```python
from build123d import *

# Parameters (mm, degrees)
ESBO_O1_W                = 170
ESBO_O1_H                = 96
RESSALTO_EXTRUS_O1_DEPTH = 6
CORTE_EXTRUS_O1_REACH    = 99.801
ESBO_O2_W                = 15.455454545
ESBO_O2_H                = 6
CORTE_EXTRUS_O2_REACH    = 99.801
ESBO_O3_W                = 6
ESBO_O3_H                = 13.714285714
CORTE_EXTRUS_O3_REACH    = 99.801
ESBO_O4_W                = 40
ESBO_O4_H                = 6
ESBO_O4_R                = 2.3
FILETE1_R                = 3


with BuildPart() as part:
    # Esboço1 → Ressalto-extrusão1 (new body)
    with BuildSketch(Plane(origin=(0, 0, 0), x_dir=(0, 0, -1), z_dir=(1, 0, 0))):
        Rectangle(ESBO_O1_W, ESBO_O1_H)
    extrude(amount=RESSALTO_EXTRUS_O1_DEPTH)

    # Esboço2 → Corte-extrusão1 (cut, up to next)
    with BuildSketch(Plane(origin=(6, 0, 0), x_dir=(0, 0, -1), z_dir=(1, 0, 0)), mode=Mode.PRIVATE) as corte_extrus_o1_sk1:
        with Locations((0.002272727, 45)):
            Rectangle(ESBO_O2_W, ESBO_O2_H)
    corte_extrus_o1_tool1 = extrude(corte_extrus_o1_sk1.sketch, amount=-CORTE_EXTRUS_O1_REACH, mode=Mode.PRIVATE) & part.part
    # Esboço2 → Corte-extrusão1 (cut, up to next)
    with BuildSketch(Plane(origin=(6, 0, 0), x_dir=(0, 0, -1), z_dir=(1, 0, 0)), mode=Mode.PRIVATE) as corte_extrus_o1_sk2:
        with Locations((-30.907727273, 45)):
            Rectangle(ESBO_O2_W, ESBO_O2_H)
    corte_extrus_o1_tool2 = extrude(corte_extrus_o1_sk2.sketch, amount=-CORTE_EXTRUS_O1_REACH, mode=Mode.PRIVATE) & part.part
    # Esboço2 → Corte-extrusão1 (cut, up to next)
    with BuildSketch(Plane(origin=(6, 0, 0), x_dir=(0, 0, -1), z_dir=(1, 0, 0)), mode=Mode.PRIVATE) as corte_extrus_o1_sk3:
        with Locations((-61.817727273, 45)):
            Rectangle(ESBO_O2_W, ESBO_O2_H)
    corte_extrus_o1_tool3 = extrude(corte_extrus_o1_sk3.sketch, amount=-CORTE_EXTRUS_O1_REACH, mode=Mode.PRIVATE) & part.part
    # Esboço2 → Corte-extrusão1 (cut, up to next)
    with BuildSketch(Plane(origin=(6, 0, 0), x_dir=(0, 0, -1), z_dir=(1, 0, 0)), mode=Mode.PRIVATE) as corte_extrus_o1_sk4:
        with Locations((30.912272728, 45)):
            Rectangle(ESBO_O2_W, ESBO_O2_H)
    corte_extrus_o1_tool4 = extrude(corte_extrus_o1_sk4.sketch, amount=-CORTE_EXTRUS_O1_REACH, mode=Mode.PRIVATE) & part.part
    # Esboço2 → Corte-extrusão1 (cut, up to next)
    with BuildSketch(Plane(origin=(6, 0, 0), x_dir=(0, 0, -1), z_dir=(1, 0, 0)), mode=Mode.PRIVATE) as corte_extrus_o1_sk5:
        with Locations((61.822272728, 45)):
            Rectangle(ESBO_O2_W, ESBO_O2_H)
    corte_extrus_o1_tool5 = extrude(corte_extrus_o1_sk5.sketch, amount=-CORTE_EXTRUS_O1_REACH, mode=Mode.PRIVATE) & part.part
    # Esboço2 → Corte-extrusão1 (cut, up to next)
    with BuildSketch(Plane(origin=(6, 0, 0), x_dir=(0, 0, -1), z_dir=(1, 0, 0)), mode=Mode.PRIVATE) as corte_extrus_o1_sk6:
        with Locations((-61.817727273, -48)):
            Rectangle(ESBO_O2_W, ESBO_O2_H)
    corte_extrus_o1_tool6 = extrude(corte_extrus_o1_sk6.sketch, amount=-CORTE_EXTRUS_O1_REACH, mode=Mode.PRIVATE) & part.part
    # Esboço2 → Corte-extrusão1 (cut, up to next)
    with BuildSketch(Plane(origin=(6, 0, 0), x_dir=(0, 0, -1), z_dir=(1, 0, 0)), mode=Mode.PRIVATE) as corte_extrus_o1_sk7:
        with Locations((-30.907727273, -48)):
            Rectangle(ESBO_O2_W, ESBO_O2_H)
    corte_extrus_o1_tool7 = extrude(corte_extrus_o1_sk7.sketch, amount=-CORTE_EXTRUS_O1_REACH, mode=Mode.PRIVATE) & part.part
    # Esboço2 → Corte-extrusão1 (cut, up to next)
    with BuildSketch(Plane(origin=(6, 0, 0), x_dir=(0, 0, -1), z_dir=(1, 0, 0)), mode=Mode.PRIVATE) as corte_extrus_o1_sk8:
        with Locations((0.002272727, -48)):
            Rectangle(ESBO_O2_W, ESBO_O2_H)
    corte_extrus_o1_tool8 = extrude(corte_extrus_o1_sk8.sketch, amount=-CORTE_EXTRUS_O1_REACH, mode=Mode.PRIVATE) & part.part
    # Esboço2 → Corte-extrusão1 (cut, up to next)
    with BuildSketch(Plane(origin=(6, 0, 0), x_dir=(0, 0, -1), z_dir=(1, 0, 0)), mode=Mode.PRIVATE) as corte_extrus_o1_sk9:
        with Locations((30.912272728, -48)):
            Rectangle(ESBO_O2_W, ESBO_O2_H)
    corte_extrus_o1_tool9 = extrude(corte_extrus_o1_sk9.sketch, amount=-CORTE_EXTRUS_O1_REACH, mode=Mode.PRIVATE) & part.part
    # Esboço2 → Corte-extrusão1 (cut, up to next)
    with BuildSketch(Plane(origin=(6, 0, 0), x_dir=(0, 0, -1), z_dir=(1, 0, 0)), mode=Mode.PRIVATE) as corte_extrus_o1_sk10:
        with Locations((61.822272728, -48)):
            Rectangle(ESBO_O2_W, ESBO_O2_H)
    corte_extrus_o1_tool10 = extrude(corte_extrus_o1_sk10.sketch, amount=-CORTE_EXTRUS_O1_REACH, mode=Mode.PRIVATE) & part.part
    add(corte_extrus_o1_tool1.solids().sort_by_distance((6, 45, -0.002273))[0], mode=Mode.SUBTRACT)
    add(corte_extrus_o1_tool2.solids().sort_by_distance((6, 45, 30.907727))[0], mode=Mode.SUBTRACT)
    add(corte_extrus_o1_tool3.solids().sort_by_distance((6, 45, 61.817727))[0], mode=Mode.SUBTRACT)
    add(corte_extrus_o1_tool4.solids().sort_by_distance((6, 45, -30.912273))[0], mode=Mode.SUBTRACT)
    add(corte_extrus_o1_tool5.solids().sort_by_distance((6, 45, -61.822273))[0], mode=Mode.SUBTRACT)
    add(corte_extrus_o1_tool6.solids().sort_by_distance((6, -48, 61.817727))[0], mode=Mode.SUBTRACT)
    add(corte_extrus_o1_tool7.solids().sort_by_distance((6, -48, 30.907727))[0], mode=Mode.SUBTRACT)
    add(corte_extrus_o1_tool8.solids().sort_by_distance((6, -48, -0.002273))[0], mode=Mode.SUBTRACT)
    add(corte_extrus_o1_tool9.solids().sort_by_distance((6, -48, -30.912273))[0], mode=Mode.SUBTRACT)
    add(corte_extrus_o1_tool10.solids().sort_by_distance((6, -48, -61.822273))[0], mode=Mode.SUBTRACT)

    # Esboço3 → Corte-extrusão2 (cut, up to next)
    with BuildSketch(Plane(origin=(6, 0, 0), x_dir=(0, 0, -1), z_dir=(1, 0, 0)), mode=Mode.PRIVATE) as corte_extrus_o2_sk1:
        with Locations((82, -41.142857143)):
            Rectangle(ESBO_O3_W, ESBO_O3_H)
    corte_extrus_o2_tool1 = extrude(corte_extrus_o2_sk1.sketch, amount=-CORTE_EXTRUS_O2_REACH, mode=Mode.PRIVATE) & part.part
    # Esboço3 → Corte-extrusão2 (cut, up to next)
    with BuildSketch(Plane(origin=(6, 0, 0), x_dir=(0, 0, -1), z_dir=(1, 0, 0)), mode=Mode.PRIVATE) as corte_extrus_o2_sk2:
        with Locations((-82, -41.142857143)):
            Rectangle(ESBO_O3_W, ESBO_O3_H)
    corte_extrus_o2_tool2 = extrude(corte_extrus_o2_sk2.sketch, amount=-CORTE_EXTRUS_O2_REACH, mode=Mode.PRIVATE) & part.part
    # Esboço3 → Corte-extrusão2 (cut, up to next)
    with BuildSketch(Plane(origin=(6, 0, 0), x_dir=(0, 0, -1), z_dir=(1, 0, 0)), mode=Mode.PRIVATE) as corte_extrus_o2_sk3:
        with Locations((82, -13.712857143)):
            Rectangle(ESBO_O3_W, ESBO_O3_H)
    corte_extrus_o2_tool3 = extrude(corte_extrus_o2_sk3.sketch, amount=-CORTE_EXTRUS_O2_REACH, mode=Mode.PRIVATE) & part.part
    # Esboço3 → Corte-extrusão2 (cut, up to next)
    with BuildSketch(Plane(origin=(6, 0, 0), x_dir=(0, 0, -1), z_dir=(1, 0, 0)), mode=Mode.PRIVATE) as corte_extrus_o2_sk4:
        with Locations((82, 13.717142857)):
            Rectangle(ESBO_O3_W, ESBO_O3_H)
    corte_extrus_o2_tool4 = extrude(corte_extrus_o2_sk4.sketch, amount=-CORTE_EXTRUS_O2_REACH, mode=Mode.PRIVATE) & part.part
    # Esboço3 → Corte-extrusão2 (cut, up to next)
    with BuildSketch(Plane(origin=(6, 0, 0), x_dir=(0, 0, -1), z_dir=(1, 0, 0)), mode=Mode.PRIVATE) as corte_extrus_o2_sk5:
        with Locations((82, 41.147142857)):
            Rectangle(ESBO_O3_W, ESBO_O3_H)
    corte_extrus_o2_tool5 = extrude(corte_extrus_o2_sk5.sketch, amount=-CORTE_EXTRUS_O2_REACH, mode=Mode.PRIVATE) & part.part
    # Esboço3 → Corte-extrusão2 (cut, up to next)
    with BuildSketch(Plane(origin=(6, 0, 0), x_dir=(0, 0, -1), z_dir=(1, 0, 0)), mode=Mode.PRIVATE) as corte_extrus_o2_sk6:
        with Locations((-82, -13.712857143)):
            Rectangle(ESBO_O3_W, ESBO_O3_H)
    corte_extrus_o2_tool6 = extrude(corte_extrus_o2_sk6.sketch, amount=-CORTE_EXTRUS_O2_REACH, mode=Mode.PRIVATE) & part.part
    # Esboço3 → Corte-extrusão2 (cut, up to next)
    with BuildSketch(Plane(origin=(6, 0, 0), x_dir=(0, 0, -1), z_dir=(1, 0, 0)), mode=Mode.PRIVATE) as corte_extrus_o2_sk7:
        with Locations((-82, 13.717142857)):
            Rectangle(ESBO_O3_W, ESBO_O3_H)
    corte_extrus_o2_tool7 = extrude(corte_extrus_o2_sk7.sketch, amount=-CORTE_EXTRUS_O2_REACH, mode=Mode.PRIVATE) & part.part
    # Esboço3 → Corte-extrusão2 (cut, up to next)
    with BuildSketch(Plane(origin=(6, 0, 0), x_dir=(0, 0, -1), z_dir=(1, 0, 0)), mode=Mode.PRIVATE) as corte_extrus_o2_sk8:
        with Locations((-82, 41.147142857)):
            Rectangle(ESBO_O3_W, ESBO_O3_H)
    corte_extrus_o2_tool8 = extrude(corte_extrus_o2_sk8.sketch, amount=-CORTE_EXTRUS_O2_REACH, mode=Mode.PRIVATE) & part.part
    add(corte_extrus_o2_tool1.solids().sort_by_distance((6, -41.142857, -82))[0], mode=Mode.SUBTRACT)
    add(corte_extrus_o2_tool2.solids().sort_by_distance((6, -41.142857, 82))[0], mode=Mode.SUBTRACT)
    add(corte_extrus_o2_tool3.solids().sort_by_distance((6, -13.712857, -82))[0], mode=Mode.SUBTRACT)
    add(corte_extrus_o2_tool4.solids().sort_by_distance((6, 13.717143, -82))[0], mode=Mode.SUBTRACT)
    add(corte_extrus_o2_tool5.solids().sort_by_distance((6, 41.147143, -82))[0], mode=Mode.SUBTRACT)
    add(corte_extrus_o2_tool6.solids().sort_by_distance((6, -13.712857, 82))[0], mode=Mode.SUBTRACT)
    add(corte_extrus_o2_tool7.solids().sort_by_distance((6, 13.717143, 82))[0], mode=Mode.SUBTRACT)
    add(corte_extrus_o2_tool8.solids().sort_by_distance((6, 41.147143, 82))[0], mode=Mode.SUBTRACT)

    # Esboço4 → Corte-extrusão3 (cut, up to next)
    with BuildSketch(Plane(origin=(6, 0, 0), x_dir=(0, 0, -1), z_dir=(1, 0, 0)), mode=Mode.PRIVATE) as corte_extrus_o3_sk1:
        with Locations((50, -4)):
            Rectangle(ESBO_O4_W, ESBO_O4_H)
    corte_extrus_o3_tool1 = extrude(corte_extrus_o3_sk1.sketch, amount=-CORTE_EXTRUS_O3_REACH, mode=Mode.PRIVATE) & part.part
    # Esboço4 → Corte-extrusão3 (cut, up to next)
    with BuildSketch(Plane(origin=(6, 0, 0), x_dir=(0, 0, -1), z_dir=(1, 0, 0)), mode=Mode.PRIVATE) as corte_extrus_o3_sk2:
        with Locations((50, -16)):
            Rectangle(ESBO_O4_W, ESBO_O4_H)
    corte_extrus_o3_tool2 = extrude(corte_extrus_o3_sk2.sketch, amount=-CORTE_EXTRUS_O3_REACH, mode=Mode.PRIVATE) & part.part
    # Esboço4 → Corte-extrusão3 (cut, up to next)
    with BuildSketch(Plane(origin=(6, 0, 0), x_dir=(0, 0, -1), z_dir=(1, 0, 0)), mode=Mode.PRIVATE) as corte_extrus_o3_sk3:
        with Locations((50, -28)):
            Rectangle(ESBO_O4_W, ESBO_O4_H)
    corte_extrus_o3_tool3 = extrude(corte_extrus_o3_sk3.sketch, amount=-CORTE_EXTRUS_O3_REACH, mode=Mode.PRIVATE) & part.part
    # Esboço4 → Corte-extrusão3 (cut, up to next)
    with BuildSketch(Plane(origin=(6, 0, 0), x_dir=(0, 0, -1), z_dir=(1, 0, 0)), mode=Mode.PRIVATE) as corte_extrus_o3_sk4:
        with Locations((30, -36)):
            Circle(ESBO_O4_R)
    corte_extrus_o3_tool4 = extrude(corte_extrus_o3_sk4.sketch, amount=-CORTE_EXTRUS_O3_REACH, mode=Mode.PRIVATE) & part.part
    # Esboço4 → Corte-extrusão3 (cut, up to next)
    with BuildSketch(Plane(origin=(6, 0, 0), x_dir=(0, 0, -1), z_dir=(1, 0, 0)), mode=Mode.PRIVATE) as corte_extrus_o3_sk5:
        with Locations((70, -36)):
            Circle(ESBO_O4_R)
    corte_extrus_o3_tool5 = extrude(corte_extrus_o3_sk5.sketch, amount=-CORTE_EXTRUS_O3_REACH, mode=Mode.PRIVATE) & part.part
    # Esboço4 → Corte-extrusão3 (cut, up to next)
    with BuildSketch(Plane(origin=(6, 0, 0), x_dir=(0, 0, -1), z_dir=(1, 0, 0)), mode=Mode.PRIVATE) as corte_extrus_o3_sk6:
        with Locations((70, 4)):
            Circle(ESBO_O4_R)
    corte_extrus_o3_tool6 = extrude(corte_extrus_o3_sk6.sketch, amount=-CORTE_EXTRUS_O3_REACH, mode=Mode.PRIVATE) & part.part
    # Esboço4 → Corte-extrusão3 (cut, up to next)
    with BuildSketch(Plane(origin=(6, 0, 0), x_dir=(0, 0, -1), z_dir=(1, 0, 0)), mode=Mode.PRIVATE) as corte_extrus_o3_sk7:
        with Locations((30, 4)):
            Circle(ESBO_O4_R)
    corte_extrus_o3_tool7 = extrude(corte_extrus_o3_sk7.sketch, amount=-CORTE_EXTRUS_O3_REACH, mode=Mode.PRIVATE) & part.part
    add(corte_extrus_o3_tool1.solids().sort_by_distance((6, -4, -50))[0], mode=Mode.SUBTRACT)
    add(corte_extrus_o3_tool2.solids().sort_by_distance((6, -16, -50))[0], mode=Mode.SUBTRACT)
    add(corte_extrus_o3_tool3.solids().sort_by_distance((6, -28, -50))[0], mode=Mode.SUBTRACT)
    add(corte_extrus_o3_tool4.solids().sort_by_distance((6, -36, -30))[0], mode=Mode.SUBTRACT)
    add(corte_extrus_o3_tool5.solids().sort_by_distance((6, -36, -70))[0], mode=Mode.SUBTRACT)
    add(corte_extrus_o3_tool6.solids().sort_by_distance((6, 4, -70))[0], mode=Mode.SUBTRACT)
    add(corte_extrus_o3_tool7.solids().sort_by_distance((6, 4, -30))[0], mode=Mode.SUBTRACT)

    # Filete1
    filete1_edges = [part.edges().sort_by_distance(p)[0] for p in [
        (3, -13, -70),
        (3, -25, -70),
        (3, -13, -30),
        (3, -25, -30),
        (3, -19, -70),
        (3, -31, -70),
        (3, -31, -30),
        (3, -19, -30),
        (3, -1, -70),
        (3, -7, -70),
        (3, -7, -30),
        (3, -1, -30),
    ]]
    fillet(filete1_edges, radius=FILETE1_R - 0.0001)  # a hair under: the kernel refuses the full size


solid = part.part
```
The model under review builds one solid part; all positions refer to its coordinate system, in mm. A direction names the side the tool comes from. Round coordinates to 2 decimals unless told otherwise and drop trailing zeros. Write each loop counter-clockwise with the first axis right and the second up, starting at its lowest first coordinate (ties: lowest second). Pieces come first, ordered by that corner, then holes.
(1) Machinability: for faces 1 (the flat face through (3, -47, -38.64)), 2 (the flat face through (3, 45, -38.64)), 3 (the flat face through (3, -20.57, 82)), which of the approach directions +Z, -Z, +X, -X, +Y, -Y give a long, thin tool a straight path to every point of the face, cutting with its end or side? Answer none if there is none.
(2) We need section D-D on z = 3. Give the boundary of the cut face in (x, y).
(3) Wall thickness on L1, parallel to Y at x = 5.2, z = -54; L2, parallel to Y at x = 2.05, z = -56; L3, parallel to Z at x = 0.45, y = 44: over which ranges is each line inside the solid? List them lowest first.
(4) We need section B-B on y = -36. Give the boundary of the cut face in (x, z).
(5) We need section A-A on y = 4. Give the boundary of the cut face in (x, z).
(6) Insertion check: pin 1 (0.9 mm diameter, centred on x = 3, y = -46.5, fed in from -Z); pin 2 (0.9 mm diameter, centred on x = 3.5, y = -46, fed in from +Z); pin 3 (3 mm diameter, centred on x = 4, z = -83, fed in from +Y). Each pin has a flat end and moves straight along its axis. Give the tip position at first contact, or say it passes through.
(7) We need section C-C on x = 5.05. Give the number of separate pieces and of enclosed holes in the cut face, and give its area (3 significant figures).
Findings below:
1. face 1: +X, -X, -Y
1. face 2: +X, -X, +Y
1. face 3: +Z, +X, -X
2. outline: (0, -45) - (6, -45) - (6, 42) - (0, 42) - close
3. L1: y = -48 to -31, -25 to -19, -13 to -7, -1 to 48
3. L2: y = -45 to -31, -25 to -19, -13 to -7, -1 to 42
3. L3: z = -79 to -69.55, -54.09 to -38.64, -23.18 to -7.73, 7.73 to 23.18, 38.64 to 54.09, 69.55 to 79
4. outline: (0, -79) - (6, -79) - (6, -72.3) - (0, -72.3) - close; (0, -67.7) - (6, -67.7) - (6, -32.3) - (0, -32.3) - close; (0, -27.7) - (6, -27.7) - (6, 79) - (0, 79) - close
5. outline: (0, -85) - (6, -85) - (6, -72.3) - (0, -72.3) - close; (0, -67.7) - (6, -67.7) - (6, -32.3) - (0, -32.3) - close; (0, -27.7) - (6, -27.7) - (6, 85) - (0, 85) - close
6. pin 1: stops at z = -79
6. pin 2: stops at z = 79
6. pin 3: stops at y = 34.29
7. separate pieces: 1
7. enclosed holes: 7
7. area: 14,200 mm2
